For this review, take the finished solid that the model builds, in its own axes (mm). A direction names the side the tool comes from. Give positions to 0.01 mm unless a question says otherwise; leave off trailing zeros. Write each loop counter-clockwise with the first axis right and the second up, starting at its lowest first coordinate (ties: lowest second). Pieces come first, ordered by that corner, then holes. Notation, with made-up numbers: M -15,25.5 L 29,25.5 A6 cw 29,35.5 Z; hole C -26.75,-39 d7. An arc over 180 degrees is marked long. One line per item, written item: value. Start each with the question number.
Item 1: Tool access review of faces 1 (the face through (-21, -1, 13)), 2 (the face through (-24, -30, 10.25)), 3 (the face through (-15.077, -12.278, 1.726)): name each direction out of +Z, -Z, +X, -X, +Y, -Y from which nothing blocks a thin tool from reaching the whole face with its end or side.
Item 2: Consider section B-B, the plane x = 0. Write out the cut boundary in (y, z).
Item 3: Consider section C-C, the plane z = 11.75. Write out the cut boundary in (x, y).
Item 4: To check wall thickness, follow probe 1 along Y at (x, z) = (-23.5, 12.75); probe 2 along X at (y, z) = (15.5, 4.3); probe 3 along Y at (x, z) = (-15.5, 5.4). State the ranges of each line that lie inside material, in increasing order.
Item 5: Consider section A-A, the plane y = 0. Write out the cut boundary in (x, z), and give its area (3 significant figures).
Item 6: Consider section D-D, the plane y = -15.5. Write out the cut boundary in (x, z), and give its area (3 significant figures).
Item 7: Clearance check with flat-ended pins moving along their axes: pin 1 Ø22 at (x, y) = (0, 0) entering from +Z; pin 2 Ø1.5 at (x, z) = (-10.5, 5) entering from +Y; pin 3 Ø5.5 at (x, y) = (15.5, 15.5) entering from -Z; pin 4 Ø6 at (x, z) = (-12.5, 8) entering from -Y. State where each tip first meets the part, or that it passes through.
Item 8: Mouldability with a two-part tool opening along Z and no side actions: class faces 4 (the face through (15.923, -12.278, 1.726)), 5 (the face through (-17, -17, 3.5)), 6 (the face through (-24, 30, 15.75)) as released by +Z, released by -Z, zero draft, split by the parting line, or undercut.
```python
from build123d import *

# Parameters (mm, degrees)
SKETCH1_R           = 12.1
SKETCH1_R_2         = 1.75
BOSS_EXTRUDE1_DEPTH = 6
SKETCH2_R           = 3.25
CUT_EXTRUDE1_DEPTH  = 3.5
FILLET2_R           = 7
SKETCH4_W           = 6
SKETCH4_H           = 80
BOSS_EXTRUDE2_DEPTH = 20
SKETCH5_W           = 5.5
SKETCH5_H           = 10
CUT_EXTRUDE2_DEPTH  = 20
FILLET3_R           = 2.75
FILLET4_R           = 6


with BuildPart() as part:
    # Sketch1 → Boss-Extrude1 (new body)
    with BuildSketch(Plane.XY):
        Polygon((21, -21), (21, 21), (-21, 40), (-21, -40), align=None)
        Circle(SKETCH1_R, mode=Mode.SUBTRACT)
        with Locations((15.5, 15.5)):
            Circle(SKETCH1_R_2, mode=Mode.SUBTRACT)
        with Locations((15.5, -15.5)):
            Circle(SKETCH1_R_2, mode=Mode.SUBTRACT)
        with Locations((-15.5, -15.5)):
            Circle(SKETCH1_R_2, mode=Mode.SUBTRACT)
        with Locations((-15.5, 15.5)):
            Circle(SKETCH1_R_2, mode=Mode.SUBTRACT)
    extrude(amount=BOSS_EXTRUDE1_DEPTH)

    # Sketch2 → Cut-Extrude1 (cut)
    with BuildSketch(Plane(origin=(0, 0, 0), x_dir=(-1, 0, 0), z_dir=(0, 0, -1))):
        with Locations((-15.5, 15.5)):
            Circle(SKETCH2_R)
        with Locations((15.5, 15.5)):
            Circle(SKETCH2_R)
        with Locations((15.5, -15.5)):
            Circle(SKETCH2_R)
        with Locations((-15.5, -15.5)):
            Circle(SKETCH2_R)
    extrude(amount=-CUT_EXTRUDE1_DEPTH, mode=Mode.SUBTRACT)

    # Fillet2
    fillet2_edges = [part.edges().sort_by_distance(p)[0] for p in [
        (21, 21, 3),
        (21, -21, 3),
    ]]
    fillet(fillet2_edges, radius=FILLET2_R)

    # Sketch4 → Boss-Extrude2 (add)
    with BuildSketch(Plane(origin=(0, 0, 0), x_dir=(-1, 0, 0), z_dir=(0, 0, -1))):
        with Locations((24, 0)):
            Rectangle(SKETCH4_W, SKETCH4_H)
    extrude(amount=-BOSS_EXTRUDE2_DEPTH)

    # Sketch5 → Cut-Extrude2 (cut)
    with BuildSketch(Plane(origin=(-21, 0, 0), x_dir=(0, 0, -1), z_dir=(1, 0, 0))):
        with Locations((-13, -30)):
            Rectangle(SKETCH5_W, SKETCH5_H)
        with Locations((-13, 30)):
            Rectangle(SKETCH5_W, SKETCH5_H)
    extrude(amount=-CUT_EXTRUDE2_DEPTH, mode=Mode.SUBTRACT)

    # Fillet3
    fillet3_edges = [part.edges().sort_by_distance(p)[0] for p in [
        (-24, -25, 15.75),
        (-24, -25, 10.25),
        (-24, -35, 15.75),
        (-24, -35, 10.25),
        (-24, 35, 15.75),
        (-24, 25, 15.75),
        (-24, 25, 10.25),
        (-24, 35, 10.25),
    ]]
    fillet(fillet3_edges, radius=FILLET3_R - 0.0001)  # a hair under: the kernel refuses the full size

    # Fillet4
    fillet4_edges = [part.edges().sort_by_distance(p)[0] for p in [
        (-24, 40, 20),
        (-24, -40, 20),
    ]]
    fillet(fillet4_edges, radius=FILLET4_R)


solid = part.part
```
Model answer:
1. face 1: +Z, +X, +Y, -Y
1. face 2: +X, -X
1. face 3: -Z
2. outline: M -30.5,0 L -12.1,0 L -12.1,6 L -30.5,6 Z; M 12.1,0 L 30.5,0 L 30.5,6 L 12.1,6 Z
3. outline: M -27,-40 L -21,-40 L -21,-34.7 L -27,-34.7 Z; M -27,-25.3 L -21,-25.3 L -21,25.3 L -27,25.3 Z; M -27,34.7 L -21,34.7 L -21,40 L -27,40 Z
4. probe 1: y = -40 to -34.99, -25.01 to 25.01, 34.99 to 40
4. probe 2: x = -27 to -17.25, -13.75 to 13.75, 17.25 to 21
4. probe 3: y = -37.51 to -17.25, -13.75 to 13.75, 17.25 to 37.51
5. outline: M -27,0 L -12.1,0 L -12.1,6 L -21,6 L -21,20 L -27,20 Z; M 12.1,0 L 21,0 L 21,6 L 12.1,6 Z
5. area: 227 mm2
6. outline: M -27,0 L -18.75,0 L -18.75,3.5 L -17.25,3.5 L -17.25,6 L -21,6 L -21,20 L -27,20 Z; M -13.75,3.5 L -12.25,3.5 L -12.25,0 L 12.25,0 L 12.25,3.5 L 13.75,3.5 L 13.75,6 L -13.75,6 Z; M 17.25,3.5 L 18.75,3.5 L 18.75,0 L 21,0 L 21,6 L 17.25,6 Z
6. area: 309 mm2
7. pin 1: passes through
7. pin 2: stops at y = 35.59
7. pin 3: stops at z = 3.5
7. pin 4: stops at y = -37.17
8. face 4: zero draft
8. face 5: released by -Z
8. face 6: undercut
